Part model, mm, in its own coordinate system. Face numbers are marked on the shaded views. A direction names the side the tool comes from. Round coordinates to 2 decimals unless told otherwise and drop trailing zeros. Loops run counter-clockwise (first coordinate to the right, second up) from the corner with the lowest first, then second, coordinate; pieces in that order, holes last.
Autodesk Inventor part; units mm, degrees
ref_plane "YZ Plane" through (0, 0, 0) normal (1, 0, 0) x (0, 1, 0)
ref_plane "XZ Plane" through (0, 0, 0) normal (0, 1, 0) x (-1, 0, 0)
ref_plane "XY Plane" through (0, 0, 0) normal (0, 0, 1) x (1, 0, 0)
sketch "Sketch1" plane through (0, 0, 0) normal (0, 1, 0) x (-1, 0, 0)
  line L0 (0, 0) -> (200, 0)
  line L1 (200, 0) -> (200, -100)
  line L2 (200, -100) -> (0, -100)
  line L3 (0, -100) -> (0, 0)
  dimension "d0" = 200
  dimension "d1" = 100
extrude "Extrusion1" add sketch "Sketch1" along normal blind 20
sketch "Sketch2" plane through (-200, 0, 0) normal (0, 0, 1) x (1, 0, 0)
  line L0 (0, 0) -> (0, 20)
  line L1 (0, 0) -> (32, 0)
  line L2 (32, 0) -> (64, 0)
  line L3 (200, 0) -> (0, 0)
  line L4 (64, 0) -> (96, 0)
  line L5 (96, 0) -> (128, 0)
  line L6 (128, 0) -> (200, 0)
  line L7 (64, 0) -> (64, 80.3945) construction
  line L8 (200, 20) -> (0, 20)
  line L9 (0, 20) -> (200, 20)
  line L10 (0, 20) -> (200, 20)
  line L11 (0, 20) -> (200, 20)
  line L12 (0, 20) -> (80, 48.5382)
  line L13 (80, 48.5382) -> (200, 20)
extrude "Extrusion2" add sketch "Sketch2" against normal blind 100
sketch "Sketch4" plane through (0, 0, 0) normal (0, -1, 0) x (1, 0, 0)
  line L0 (0, 0) -> (-5, 0)
  line L1 (-5, 0) -> (-5, -5)
  line L2 (-5, -5) -> (0, -5)
  line L3 (0, -5) -> (0, 0)
  line L4 (-120, 0) -> (-120, -100)
  line L5 (-120, 0) -> (-115, 0)
  line L6 (-115, 0) -> (-115, -5)
  line L7 (-115, -5) -> (-120, -5)
  line L8 (-120, -5) -> (-120, 0)
  line L9 (-120, -100) -> (-115, -100)
  line L10 (-115, -100) -> (-115, -95)
  line L11 (-115, -95) -> (-120, -95)
  line L12 (-120, -95) -> (-120, -100)
  line L13 (-115, -5) -> (-5, -5)
  line L14 (-5, -5) -> (-5, -95)
  line L15 (-5, -95) -> (-115, -95)
  line L16 (-115, -95) -> (-115, -5)
  dimension "d23" = 5
  dimension "d24" = 5
  dimension "d25" = 5
  dimension "d26" = 5
  dimension "d27" = 5
  dimension "d28" = 5
extrude "Extrusion3" cut sketch "Sketch4" against normal blind 68.75 contours L14 L15 L16 L13
extrude "Extrusion4" add sketch "Sketch4" against normal blind 10 contours L14 L15 L16 L13
properties part number "Cybertruck 1"
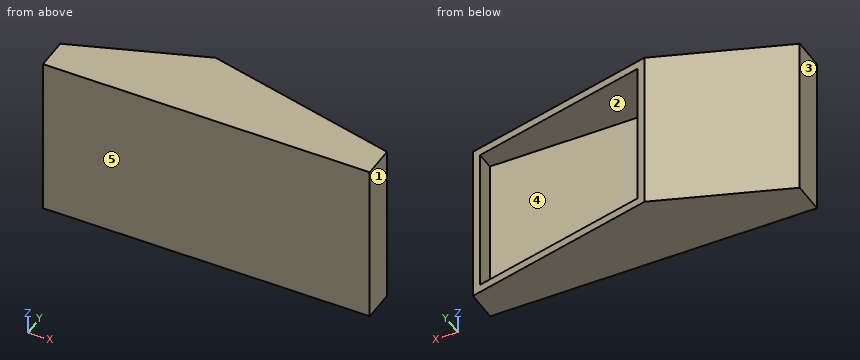
1) Slice it at A-A, the plane y = 13. Give the cut face in (x, z), then the cut area to 3 significant figures.
Values:
outline: (-200, -100) - (0, -100) - (0, 0) - (-200, 0) - close; hole (-115, -95) - (-5, -95) - (-5, -5) - (-115, -5) - close
area: 10,100 mm2
2) Mould opens along X. For the marked faces 1, 2 and 3 say: released by +X, released by -X, zero draft, split by the parting line, or undercut.
Values:
face 1: released by +X
face 2: undercut
face 3: released by -X
3) Drop flat-ended pins along their axis: pin 1 Ø8 at (x, z) = (-161.5, -87) entering from +Y; pin 2 Ø3 at (x, z) = (-97.5, -13) entering from +Y. Give the stop position or say it passes through.
Values:
pin 1: stops at y = 35.16
pin 2: stops at y = 10
4) Slice it at C-C, the plane x = -12.5. Give the cut face in (y, z), then the cut area to 3 significant figures.
Values:
outline: (0, -100) - (22.97, -100) - (22.97, -95) - (10, -95) - (10, -5) - (22.97, -5) - (22.97, 0) - (0, 0) - close
area: 1,130 mm2
5) Slice it at D-D, the plane y = 40. Give the cut face in (x, z).
Values:
outline: (-143.93, -100) - (-84.1, -100) - (-84.1, -95) - (-115, -95) - (-115, -5) - (-84.1, -5) - (-84.1, 0) - (-143.93, 0) - close
6) Slice it at B-B, the plane z = -57.5. Give the cut face in (x, y).
Values:
outline: (-200, 0) - (0, 0) - (0, 20) - (-5, 21.19) - (-5, 10) - (-115, 10) - (-115, 47.35) - (-120, 48.54) - (-200, 20) - close
7) Tool access for the marked faces 4 and 5: list every direction of +Z, -Z, +X, -X, +Y, -Y with a clear straight run to the whole face (end or side of a thin tool).
Values:
face 4: +Y
face 5: +Z, -Z, +X, -X, -Y
8) Wall check: line 1 along X through (y, z) = (15.5, -70.5); line 2 along Z through (x, y) = (-96, 38); line 3 along Y through (x, z) = (-105.5, -38.5). Give the ranges that are in metal, low to high.
Values:
line 1: x = -200 to -115, -5 to 0
line 2: z = -100 to -95, -5 to 0
line 3: y = 0 to 10
